Check sheet for the modelled part. Datum: model origin and axes. Units: mm. Face numbers are marked on the shaded views. Round coordinates to 2 decimals unless told otherwise and drop trailing zeros. Write each loop counter-clockwise with the first axis right and the second up, starting at its lowest first coordinate (ties: lowest second). Pieces come first, ordered by that corner, then holes. Notation, with made-up numbers: M -11.5,75.5 L -3.5,75.5 A27 cw -3.5,104.5 Z; hole C -22,-13.5 d10. An arc over 180 degrees is marked long. Answer in a Markdown table with one row per item.
```python
from build123d import *

# Parameters (mm, degrees)
SKETCH1_R           = 4
BOSS_EXTRUDE1_DEPTH = 6.5
CHAMFER1_SIZE       = 0.65


with BuildPart() as part:
    # Sketch1 → Boss-Extrude1 (new body)
    with BuildSketch(Plane(origin=(0, 0, 0), x_dir=(1, 0, 0), z_dir=(0, 1, 0))):
        Polygon((7.505553499, 0), (3.75277675, 6.5), (-3.75277675, 6.5), (-7.505553499, 0), (-3.75277675, -6.5), (3.75277675, -6.5), align=None)
        with Locations(Location((0, 0, 0), (0, 0, 90))):
            Circle(SKETCH1_R, mode=Mode.SUBTRACT)
    extrude(amount=BOSS_EXTRUDE1_DEPTH)

    # Sketch3 → Cut-Revolve1 (revolve, cut)
    with BuildSketch(Plane(origin=(0, 0, 0), x_dir=(0, 0, -1), z_dir=(1, 0, 0))):
        Polygon((-6.5, 0), (-8.75, 2.25), (-8.75, 0), align=None)
        Polygon((-8.75, 6.5), (-6.5, 6.5), (-8.75, 4.25), align=None)
    revolve(axis=Axis((0, 0, 0), (0, 1, 0)), mode=Mode.SUBTRACT)

    # Chamfer1
    chamfer1_edges = [part.edges().sort_by_distance(p)[0] for p in [
        (0, 0, 4),
        (0, 6.5, 4),
    ]]
    chamfer(chamfer1_edges, length=CHAMFER1_SIZE)


solid = part.part
```
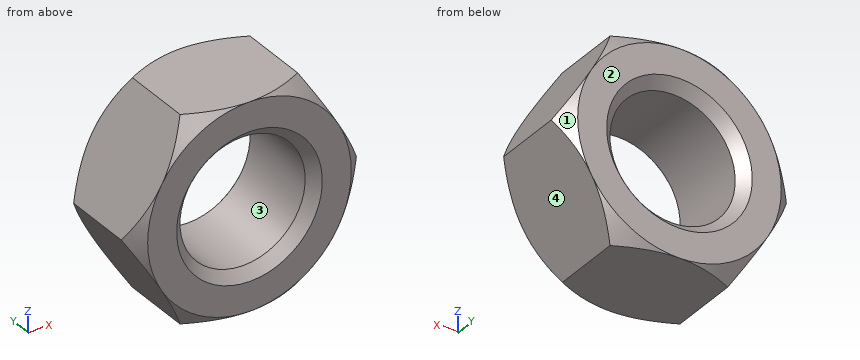
1. Go/stop test with flat-tipped pins: pin 1 (1.5 mm diameter, centred on x = -5.5, z = -2.5, fed in from -Y); pin 2 (7 mm diameter, centred on x = 0, z = 0, fed in from +Y). Record where each tip stops, or that it passes through.
Found:
| item | result |
|---|---|
| pin 1 | stops at y = 0 |
| pin 2 | passes through |
2. Scan lines: L1, parallel to Z at x = 1.25, y = 1.5; L2, parallel to Z at x = -0.5, y = 6.25; L3, parallel to X at y = 3.75, z = -0.5. Record each from-to range of solid material in increasing order.
Found:
| item | result |
|---|---|
| L1 | z = -6.5 to -3.8, 3.8 to 6.5 |
| L2 | z = -6.5 to -4.37, 4.37 to 6.5 |
| L3 | x = -7.22 to -3.97, 3.97 to 7.22 |
3. Section check A-A, the plane y = 4.75. Record the cut outline in (x, z).
Found:
| item | result |
|---|---|
| outline | M -7.51,0 L -3.75,-6.5 L 3.75,-6.5 L 7.51,0 L 3.75,6.5 L -3.75,6.5 Z; hole C 0,0 d8 |
4. Draft check along Z on the marked faces 1, 2, 3 and 4. Enter one of: +Z half, -Z half, draft (parallel to the pull), parting line (faces both ways), or undercut.
Found:
| item | result |
|---|---|
| face 1 | parting line |
| face 2 | draft |
| face 3 | undercut |
| face 4 | -Z half |
5. Section check B-B, the plane y = 6.25. Record the cut outline in (x, z), and give its area (3 significant figures).
Found:
| item | result |
|---|---|
| outline | M -6.54,-1.67 L -4.72,-4.83 A6.75 ccw -1.82,-6.5 L 1.82,-6.5 A6.75 ccw 4.72,-4.83 L 6.54,-1.67 A6.75 ccw 6.54,1.67 L 4.72,4.83 A6.75 ccw 1.82,6.5 L -1.82,6.5 A6.75 ccw -4.72,4.83 L -6.54,1.67 A6.75 ccw Z; hole C 0,0 d8.8 |
| area | 78.7 mm2 |
